Work out the finished part from the listing and answer in its coordinate system (mm). Face numbers are marked on the shaded views. A direction names the side the tool comes from. Give positions to 0.01 mm unless a question says otherwise; leave off trailing zeros. Loops run counter-clockwise (first coordinate to the right, second up) from the corner with the lowest first, then second, coordinate; pieces in that order, holes last. Notation, with made-up numbers: (-3.5, -10) - (2.5, -10) arc R16 ccw to (2.5, 4) - close; hole circle Ø2 at (89.5, 73.25). An arc over 180 degrees is marked (long way). One line per question, with ' | ' between items.
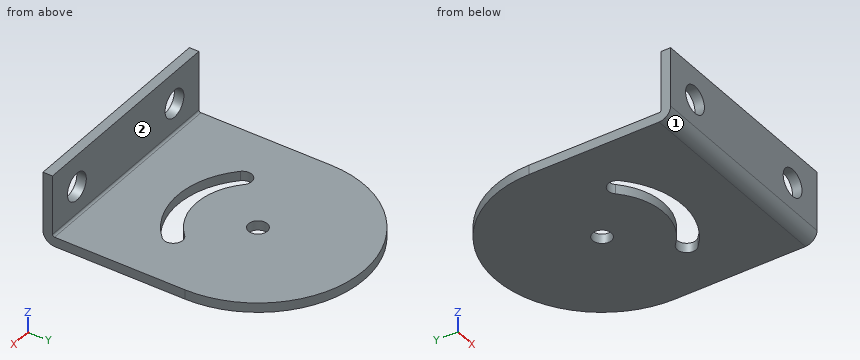
from build123d import *

# Parameters (mm, degrees)
BASE_FLANGE1_DEPTH                = 3.4036
EDGE_FLANGE2_STRIP_W              = 15.0876
EDGE_FLANGE2_STRIP_H              = 3.4036
EDGE_FLANGE2_STRIP_CUT_DEPTH      = 76.2
EDGE_FLANGE2_DEPTH                = 76.2
F_1_4_START                       = -50.8
F_1_4_CLEARANCE_HOLE3_OUTLINE_R   = 4.9022
F_1_4_CLEARANCE_HOLE3_DEPTH       = 3.4036
F_1_4_START_2                     = -3.4036
F_1_4_CLEARANCE_HOLE3_2_OUTLINE_R = 3.3782
F_1_4_CLEARANCE_HOLE3_2_DEPTH     = 3.4036
CUT_EXTRUDE1_DEPTH                = 95.185570089


# Read off the part's stored shape, not the designer's step: 1/4 Clearance Hole3
# Sheet-metal steps are written as plain solids
with BuildPart() as part:
    # Sketch1 → Base-Flange1 (new body)
    with BuildSketch(Plane.XY):
        with BuildLine():
            Line((0, 0), (0, -50.8))
            Line((0, -50.8), (-76.2, -50.8))
            Line((-76.2, -50.8), (-76.2, 0))
            ThreePointArc((-76.2, 0), (-38.1, 38.1), (0, 0))
        make_face()
    extrude(amount=-BASE_FLANGE1_DEPTH)

    # Edge-Flange2 strip (across the edge) → Edge-Flange2 strip cut (cut)
    with BuildSketch(Plane(origin=(-76.2, -50.8, 0), x_dir=(0, 1, 0), z_dir=(1, 0, 0))):
        with Locations((-3.4036, -1.7018)):
            Rectangle(EDGE_FLANGE2_STRIP_W, EDGE_FLANGE2_STRIP_H)
    extrude(amount=EDGE_FLANGE2_STRIP_CUT_DEPTH, mode=Mode.SUBTRACT)

    # Edge-Flange2 section (across the edge) → Edge-Flange2 (add)
    with BuildSketch(Plane(origin=(-76.2, -50.8, 0), x_dir=(0, 1, 0), z_dir=(1, 0, 0))):
        with BuildLine():
            Line((0, 0.7366), (0, 21.9964))
            Line((0, 21.9964), (3.4036, 21.9964))
            Line((3.4036, 21.9964), (3.4036, 0.7366))
            ThreePointArc((3.4036, 0.7366), (3.619345145, 0.215745145), (4.1402, 0))
            Line((4.1402, 0), (4.1402, -3.4036))
            ThreePointArc((4.1402, -3.4036), (1.212636505, -2.190963495), (0, 0.7366))
        make_face()
    extrude(amount=EDGE_FLANGE2_DEPTH)

    # 1/4 Clearance Hole3 outline → 1/4 Clearance Hole3 (cut)
    with BuildSketch(Plane(origin=(0, 0, 0), x_dir=(1, 0, 0), z_dir=(0, 1, 0)).offset(F_1_4_START)):
        with Locations((-12.7, -10.5664)):
            Circle(F_1_4_CLEARANCE_HOLE3_OUTLINE_R)
        with Locations((-63.5, -10.5664)):
            Circle(F_1_4_CLEARANCE_HOLE3_OUTLINE_R)
    extrude(amount=F_1_4_CLEARANCE_HOLE3_DEPTH, mode=Mode.SUBTRACT)

    # 1_4 Clearance Hole3 2 outline → 1_4 Clearance Hole3 2 (cut)
    with BuildSketch(Plane.XY.offset(F_1_4_START_2)):
        with Locations((-38.1, 0)):
            Circle(F_1_4_CLEARANCE_HOLE3_2_OUTLINE_R)
    extrude(amount=F_1_4_CLEARANCE_HOLE3_2_DEPTH, mode=Mode.SUBTRACT)

    # Sketch25 → Cut-Extrude1 (cut, through all)
    with BuildSketch(Plane.XY):
        with BuildLine():
            ThreePointArc((-58.447600474, -20.347600474), (-38.1, -28.775852552), (-17.752399526, -20.347600474))
            ThreePointArc((-17.752399526, -20.347600474), (-17.752399526, -15.570104217), (-22.529895783, -15.570104217))
            ThreePointArc((-22.529895783, -15.570104217), (-38.1, -22.019452552), (-53.670104217, -15.570104217))
            ThreePointArc((-53.670104217, -15.570104217), (-58.447600474, -15.570104217), (-58.447600474, -20.347600474))
        make_face()
    extrude(amount=-CUT_EXTRUDE1_DEPTH, mode=Mode.SUBTRACT)


solid = part.part
1. Flat-ended cylindrical pins translate along their axes: pin 1 (1.5 mm diameter, centred on x = -43.5, y = 25, fed in from +Z); pin 2 (2 mm diameter, centred on x = -58.5, y = -19, fed in from -Z). Find the tip coordinate at first contact, or state that the pin passes through.
Evaluation:
pin 1: z = 0 | pin 2: z = -3.4
2. Consider L1, parallel to Y at x = -38.1, z = -1.9; L2, parallel to Z at x = -49, y = 26; L3, parallel to Z at x = -12.7, y = -48.2. Determine where each line is inside the solid, lowest interval first.
Evaluation:
L1: -49.85 to -28.78, -22.02 to -3.38, 3.38 to 38.1 | L2: -3.4 to 0 | L3: -3.11 to 5.66, 15.47 to 22
3. Find section D-D on z = -1.75. Write down the section's boundary in (x, y), then the cut area to 3 significant figures.
Evaluation:
outline: (-76.2, -49.97) - (0, -49.97) - (0, 0) arc R38.1 ccw to (-76.2, 0) - close; hole (-58.45, -20.35) arc R28.78 ccw to (-17.75, -20.35) arc R3.38 ccw to (-22.53, -15.57) arc R22.02 cw to (-53.67, -15.57) arc R3.38 ccw to start; hole circle Ø6.76 at (-38.1, 0) | area: 5,750 mm2
4. Find section C-C on x = -10.5. Write down the section's boundary in (y, z) (3 decimals), then the cut area to 3 significant figures.
Evaluation:
outline: (-50.8, 0.737) arc R4.14 ccw to (-46.66, -3.404) - (26.265, -3.404) - (26.265, 0) - (-46.66, 0) arc R0.737 cw to (-47.396, 0.737) - (-47.396, 6.186) - (-50.8, 6.186) - close; (-50.8, 14.947) - (-47.396, 14.947) - (-47.396, 21.996) - (-50.8, 21.996) - close | area: 304 mm2
5. Find section B-B on z = 8.5. Write down the section's boundary in (x, y).
Evaluation:
outline: (-76.2, -50.8) - (-67.95, -50.8) - (-67.95, -47.4) - (-76.2, -47.4) - close; (-59.05, -50.8) - (-17.15, -50.8) - (-17.15, -47.4) - (-59.05, -47.4) - close; (-8.25, -50.8) - (0, -50.8) - (0, -47.4) - (-8.25, -47.4) - close
6. Find section A-A on x = -38.1. Write down the section's boundary in (y, z).
Evaluation:
outline: (-50.8, 0.74) arc R4.14 ccw to (-46.66, -3.4) - (-28.78, -3.4) - (-28.78, 0) - (-46.66, 0) arc R0.74 cw to (-47.4, 0.74) - (-47.4, 22) - (-50.8, 22) - close; (-22.02, -3.4) - (-3.38, -3.4) - (-3.38, 0) - (-22.02, 0) - close; (3.38, -3.4) - (38.1, -3.4) - (38.1, 0) - (3.38, 0) - close
7. Which of the six approach directions +Z, -Z, +X, -X, +Y, -Y give full straight-line access (tool end or side, diameter ignored) to the marked faces 1 and 2?
Evaluation:
face 1: -Z, +X, -X, -Y | face 2: +Z, +X, -X, +Y
